Answer from the drawing. Dimensions are ordinates in mm from the lowest x, y and z of the part. Round coordinates to 2 decimals unless told otherwise and drop trailing zeros. Order: outer loops, then holes, each group sorted by start corner. A loop starts at its lowest first (then second) coordinate and runs counter-clockwise, first axis right, second up.
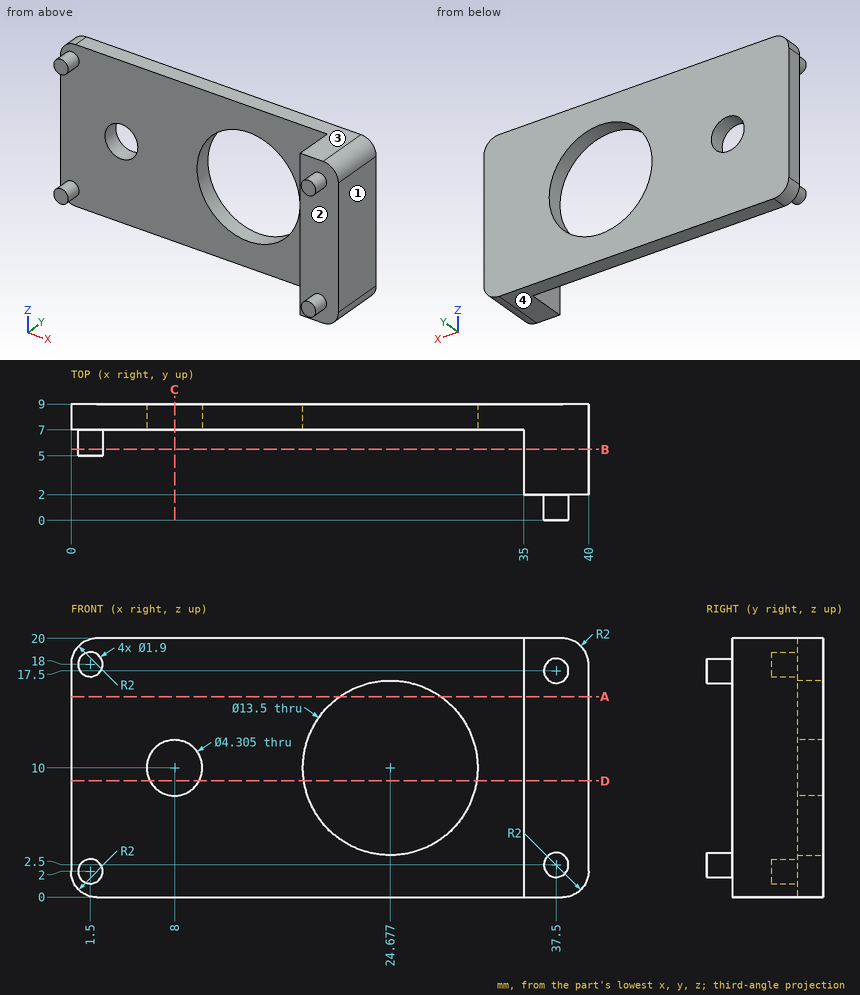
Q1. A cutting plane is placed at A-A, the plane z = 15.5. Give the vertices of the cut face in (x, y), plus the area to 3 significant figures.
Outcome:
outline: (0, 7) - (20.76, 7) - (20.76, 9) - (0, 9) - close; (28.59, 7) - (35, 7) - (35, 2) - (40, 2) - (40, 9) - (28.59, 9) - close
area: 89.3 mm2
Q2. A cutting plane is placed at D-D, the plane z = 9. Give the vertices of the cut face in (x, y), plus the area to 3 significant figures.
Outcome:
outline: (0, 7) - (6.09, 7) - (6.09, 9) - (0, 9) - close; (9.91, 7) - (18, 7) - (18, 9) - (9.91, 9) - close; (31.35, 7) - (35, 7) - (35, 2) - (40, 2) - (40, 9) - (31.35, 9) - close
area: 70.7 mm2
Q3. A cutting plane is placed at C-C, the plane x = 8. Give the vertices of the cut face in (y, z), plus the area to 3 significant figures.
Outcome:
outline: (7, 0) - (9, 0) - (9, 7.85) - (7, 7.85) - close; (7, 12.15) - (9, 12.15) - (9, 20) - (7, 20) - close
area: 31.4 mm2
Q4. Straight lines are drawn through the part: probe 1 along X at (y, z) = (7.85, 10); probe 2 along Z at (x, y) = (8, 7.85); probe 3 along Y at (x, z) = (37, 1.5). For each, find the intervals that lie inside material, in ascending order.
Outcome:
probe 1: x = 0 to 5.85, 10.15 to 17.93, 31.43 to 40
probe 2: z = 0 to 7.85, 12.15 to 20
probe 3: y = 2 to 9
Q5. A cutting plane is placed at B-B, the plane y = 5.5. Give the vertices of the cut face in (x, z).
Outcome:
outline: circle Ø1.9 at (1.5, 2); circle Ø1.9 at (1.5, 18); (35, 0) - (38, 0) arc R2 ccw to (40, 2) - (40, 18) arc R2 ccw to (38, 20) - (35, 20) - close
Q6. Flat-ended cylindrical pins translate along their axes: pin 1 (0.9 mm diameter, centred on x = 1, z = 18, fed in from -Y); pin 2 (4 mm diameter, centred on x = 37, z = 15, fed in from -Y); pin 3 (1.5 mm diameter, centred on y = 5, z = 6, fed in from -X); pin 4 (6 mm diameter, centred on x = 4, z = 11.5, fed in from -Y). Find the tip coordinate at first contact, or state that the pin passes through.
Outcome:
pin 1: stops at y = 5
pin 2: stops at y = 0
pin 3: stops at x = 35
pin 4: stops at y = 7
Q7. For a pull along Z with two mould halves and no side action, classify the marked faces 1, 2, 3 and 4 as released by +Z, released by -Z, zero draft, split by the parting line, or undercut.
Outcome:
face 1: zero draft
face 2: undercut
face 3: released by +Z
face 4: released by -Z
